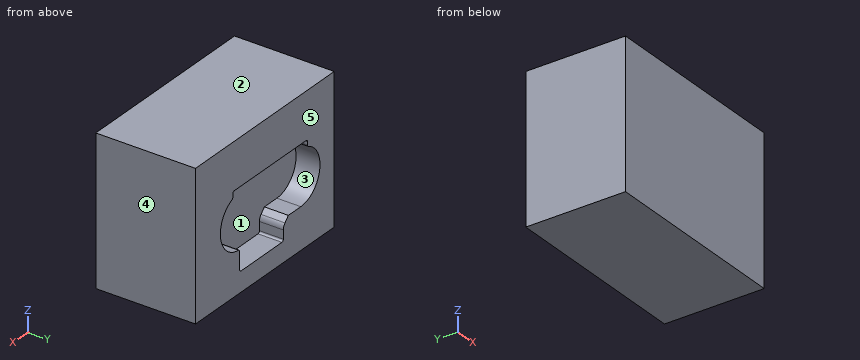
```python
from build123d import *

# Parameters (mm, degrees)
SKETCH1_W           = 290
SKETCH1_H           = 400
BOSS_EXTRUDE1_DEPTH = 35
SKETCH2_W           = 270
SKETCH2_H           = 380
CUT_EXTRUDE2_DEPTH  = 10
CUT_EXTRUDE3_DEPTH  = 6
FILLET2_R           = 2
FILLET4_R           = 0.5
FILLET5_R           = 0.5
FILLET6_R           = 0.5
FILLET7_R           = 0.5
FILLET8_R           = 0.5
FILLET9_R           = 0.5
SKETCH4_W           = 290
SKETCH4_H           = 400
SKETCH4_W_2         = 48.749470761
SKETCH4_H_2         = 36.632728687
CUT_EXTRUDE4_DEPTH  = 250.499498997


with BuildPart() as part:
    # Sketch1 → Boss-Extrude1 (new body)
    with BuildSketch(Plane(origin=(0, 0, 0), x_dir=(1, 0, 0), z_dir=(0, 1, 0))):
        Rectangle(SKETCH1_W, SKETCH1_H)
    extrude(amount=BOSS_EXTRUDE1_DEPTH)

    # Sketch2 → Cut-Extrude2 (cut)
    with BuildSketch(Plane(origin=(0, 35, 0), x_dir=(1, 0, 0), z_dir=(0, 1, 0))):
        Rectangle(SKETCH2_W, SKETCH2_H)
    extrude(amount=-CUT_EXTRUDE2_DEPTH, mode=Mode.SUBTRACT)

    # Sketch3 → Cut-Extrude3 (cut)
    with BuildSketch(Plane(origin=(0, 25, 0), x_dir=(1, 0, 0), z_dir=(0, 1, 0))):
        with BuildLine():
            Line((-117.13, 185), (-101.75, 185))
            Line((-101.75, 185), (-101.75, 179.7))
            ThreePointArc((-101.75, 179.7), (-95.105829623, 174.14058809), (-99.406157002, 166.62))
            Line((-99.406157002, 166.62), (-99.406157002, 165))
            Line((-99.406157002, 165), (-125.593842998, 165))
            Line((-125.593842998, 165), (-125.593842998, 166.62))
            ThreePointArc((-125.593842998, 166.62), (-129.894170377, 174.14058809), (-123.25, 179.7))
            Line((-123.25, 179.7), (-118.879314151, 179.7))
            Line((-118.879314151, 179.7), (-117.13, 181.5))
            Line((-117.13, 181.5), (-117.13, 185))
        make_face()
    extrude(amount=-CUT_EXTRUDE3_DEPTH, mode=Mode.SUBTRACT)

    # Fillet2
    fillet2_edges = [part.edges().sort_by_distance(p)[0] for p in [
        (-117.13, 22, -181.5),
    ]]
    fillet(fillet2_edges, radius=FILLET2_R)

    # Fillet4
    fillet4_edges = [part.edges().sort_by_distance(p)[0] for p in [
        (-125.593842998, 22, -166.62),
    ]]
    fillet(fillet4_edges, radius=FILLET4_R)

    # Fillet5
    fillet5_edges = [part.edges().sort_by_distance(p)[0] for p in [
        (-99.406157002, 22, -166.62),
    ]]
    fillet(fillet5_edges, radius=FILLET5_R)

    # Fillet6
    fillet6_edges = [part.edges().sort_by_distance(p)[0] for p in [
        (-101.75, 22, -179.7),
    ]]
    fillet(fillet6_edges, radius=FILLET6_R)

    # Fillet7
    fillet7_edges = [part.edges().sort_by_distance(p)[0] for p in [
        (-101.75, 22, -185),
    ]]
    fillet(fillet7_edges, radius=FILLET7_R)

    # Fillet8
    fillet8_edges = [part.edges().sort_by_distance(p)[0] for p in [
        (-117.13, 22, -185),
    ]]
    fillet(fillet8_edges, radius=FILLET8_R)

    # Fillet9
    fillet9_edges = [part.edges().sort_by_distance(p)[0] for p in [
        (-99.406157002, 22, -165),
        (-125.593842998, 22, -165),
    ]]
    fillet(fillet9_edges, radius=FILLET9_R)

    # Sketch4 → Cut-Extrude4 (cut, through all)
    with BuildSketch(Plane(origin=(0, 35, 0), x_dir=(1, 0, 0), z_dir=(0, 1, 0))):
        Rectangle(SKETCH4_W, SKETCH4_H)
        with Locations((-110.62526462, 171.683635657)):
            Rectangle(SKETCH4_W_2, SKETCH4_H_2, mode=Mode.SUBTRACT)
    extrude(amount=-CUT_EXTRUDE4_DEPTH, mode=Mode.SUBTRACT)


solid = part.part
```
Here's how the part is built. I have some questions about the finished solid (model axes, mm). Face numbers are marked on the shaded views. A direction names the side the tool comes from. Round coordinates to 2 decimals unless told otherwise and drop trailing zeros. Order: outer loops, then holes, each group sorted by start corner. A loop starts at its lowest first (then second) coordinate and runs counter-clockwise, first axis right, second up. Notation, with made-up numbers: M 25,70.5 L 72,70.5 A32 cw 72,97.5 Z; hole C -26.5,16 d8. An arc over 180 degrees is marked long. Answer in a Markdown table with one row per item.
Item 1: For the marked faces 1 and 2, which set-ups out of +Z, -Z, +X, -X, +Y, -Y let a thin tool reach every point of the face, with its end or its side?
A:
| item | result |
|---|---|
| face 1 | +Y |
| face 2 | +Z, +X, -X, +Y, -Y |
Item 2: If I drill on L1, parallel to Z at x = -119.5, y = 24; L2, parallel to X at y = 23.75, z = -176.5; L3, parallel to X at y = 23.75, z = -170, over which ranges is the centre line in solid material (lowest first)? Write a range as from..to.
A:
| item | result |
|---|---|
| L1 | z = -190..-179.7, -165..-153.37 |
| L2 | x = -135..-128.99, -96.01..-86.25 |
| L3 | x = -135..-129.32, -95.68..-86.25 |
Item 3: Thinking about a two-plate mould opening in X: for the marked faces 3, 4 and 5, which applies, +X half, -X half, draft (parallel to the pull), parting line (faces both ways), or undercut?
A:
| item | result |
|---|---|
| face 3 | undercut |
| face 4 | +X half |
| face 5 | draft |
Item 4: Imagine slicing it at C-C, the plane x = -119.5. Write out the boundary of the cut face in (y, z).
A:
| item | result |
|---|---|
| outline | M 0,-190 L 25,-190 L 25,-179.7 L 19,-179.7 L 19,-165 L 25,-165 L 25,-153.37 L 0,-153.37 Z |
Item 5: Imagine slicing it at A-A, the plane z = -177. Write out the boundary of the cut face in (x, y), and give its area (3 significant figures).
A:
| item | result |
|---|---|
| outline | M -135,0 L -86.25,0 L -86.25,25 L -96.35,25 L -96.35,19 L -128.65,19 L -128.65,25 L -135,25 Z |
| area | 1,020 mm2 |
Item 6: I'm going to push a flat-ended pin straight in: pin 1 (6 mm diameter, centred on x = -105, z = -170, fed in from +Y). Where does the tip first touch, or does it pass through?
A:
| item | result |
|---|---|
| pin 1 | stops at y = 19 |
Item 7: Imagine slicing it at B-B, the plane y = 22.5. Write out the boundary of the cut face in (x, z).
A:
| item | result |
|---|---|
| outline | M -135,-190 L -86.25,-190 L -86.25,-153.37 L -135,-153.37 Z; hole M -125.9,-166.74 A6.75 ccw -123.25,-179.7 L -118.88,-179.7 L -117.7,-180.92 A2 cw -117.13,-182.31 L -117.13,-184.5 A0.5 ccw -116.63,-185 L -102.25,-185 A0.5 ccw -101.75,-184.5 L -101.75,-180.18 A0.5 cw -101.28,-179.68 A6.75 ccw -99.1,-166.74 A0.5 cw -99.41,-166.28 L -99.41,-165.5 A0.5 ccw -99.91,-165 L -125.09,-165 A0.5 ccw -125.59,-165.5 L -125.59,-166.28 A0.5 cw Z |
